Read the model definition and answer for the solid it produces. Units are mm, in the model's axes. Coordinates: 2 decimals unless noted, no trailing zeros. Write each loop counter-clockwise with the first axis right and the second up, starting at its lowest first coordinate (ties: lowest second). Pieces come first, ordered by that corner, then holes.
(1) The part is cut by section C-C, the plane x = 70.5. Determine the outline of the cut face in (y, z), and give its area (3 significant figures).
(2) Straight lines are drawn through the part: line 1 along Z through (x, y) = (21, 0); line 2 along Z through (x, y) = (24, 21.5); line 3 along Y through (x, z) = (13.5, 22). For each, find the intervals that lie inside material, in ascending order.
(3) Given pin 1 (1 mm diameter, centred on x = 20.5, y = 41, fed in from -Z); pin 2 (1 mm diameter, centred on x = 48, z = -2, fed in from +Y); pin 3 (2 mm diameter, centred on x = 57.5, y = 20, fed in from -Z), each flat-ended and moving along its own axis, determine where each tip first touches the part or whether it passes through.
(4) The part is cut by section D-D, the plane x = 44. Determine the outline of the cut face in (y, z).
(5) The part is cut by section A-A, the plane z = 0. Determine the outline of the cut face in (x, y).
```python
from build123d import *

# Parameters (mm, degrees)
F0_R     = 75
F1_DEPTH = 80
F2_R     = 25
F3_DEPTH = 100
F4_R     = 35


with BuildPart() as f1:
    # F0 (on Right) → F1 (new body)
    with BuildSketch(Plane.YZ):
        Circle(F0_R)
    extrude(amount=F1_DEPTH)

    # F2 (on face) → F3 (cut)
    with BuildSketch(Plane(origin=(0, 0, 0), x_dir=(0, -1, 0), z_dir=(-1, 0, 0))):
        Circle(F2_R)
    extrude(amount=-F3_DEPTH, mode=Mode.SUBTRACT)

    # F4 (on Top) → F5 (revolve, cut)
    with BuildSketch(Plane.XY):
        with Locations((40, -75)):
            Circle(F4_R)
    revolve(axis=Axis((0, 0, 0), (-1, 0, 0)), mode=Mode.SUBTRACT)


solid = f1.part
```
Computed:
1. outline: circle Ø115.66 at (0, 0); hole circle Ø50 at (0, 0)
1. area: 8,540 mm2
2. line 1: z = -45.61 to -25, 25 to 45.61
2. line 2: z = -38.24 to -12.76, 12.76 to 38.24
2. line 3: y = -47.27 to -11.87, 11.87 to 47.27
3. pin 1: stops at z = -21.92
3. pin 2: stops at y = 41
3. pin 3: stops at z = -40.79
4. outline: circle Ø80.46 at (0, 0); hole circle Ø50 at (0, 0)
5. outline: (0, -75) - (5, -75) arc R35 cw to (75, -75) - (80, -75) - (80, -25) - (0, -25) - close; (0, 25) - (80, 25) - (80, 75) - (75, 75) arc R35 cw to (5, 75) - (0, 75) - close
